Here's how the part is built. I have some questions about the finished solid (model axes, mm). Face numbers are marked on the shaded views. A direction names the side the tool comes from. Give positions to 0.01 mm unless a question says otherwise; leave off trailing zeros. Order: outer loops, then holes, each group sorted by start corner. A loop starts at its lowest first (then second) coordinate and runs counter-clockwise, first axis right, second up.
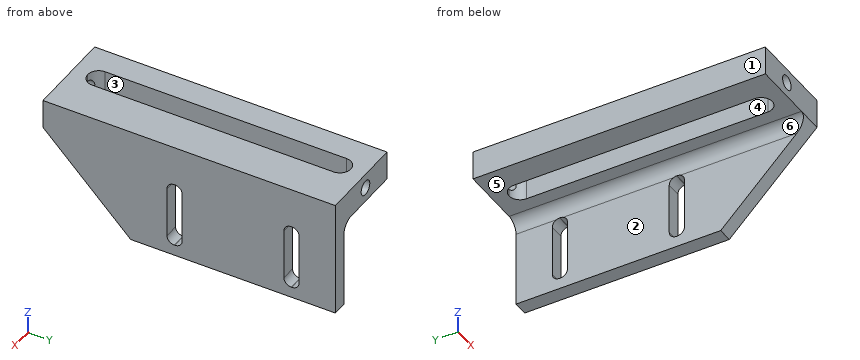
from build123d import *

# Parameters (mm, degrees)
F1_DEPTH  = 127
F2_R      = 5.08
F4_DEPTH  = 50.801
F5_R      = 3.175
F6_DEPTH  = 127.001
F8_DEPTH  = 38.101
F10_DEPTH = 38.101


with BuildPart() as f1:
    # F0 (on Front) → F1 (new body)
    with BuildSketch(Plane.XZ):
        Polygon((19.05, -25.4), (19.05, 25.4), (-19.05, 25.4), (-19.05, 12.7), (12.7, 12.7), (12.7, -25.4), align=None)
    extrude(amount=F1_DEPTH)

    # F2
    f2_edges = [f1.edges().sort_by_distance(p)[0] for p in [
        (12.7, -63.5, 12.7),
    ]]
    fillet(f2_edges, radius=F2_R)

    # F3 (on face) → F4 (cut, through all)
    with BuildSketch(Plane.XY.offset(25.4)):
        with BuildLine():
            Line((-3.1623, -6.35), (-3.1877, -6.35))
            ThreePointArc((-3.1877, -6.35), (-6.546316, -7.741184), (-7.9375, -11.0998))
            Line((-7.9375, -11.0998), (-7.9375, -115.9002))
            ThreePointArc((-7.9375, -115.9002), (-6.546316, -119.258816), (-3.1877, -120.65))
            Line((-3.1877, -120.65), (-3.1623, -120.65))
            ThreePointArc((-3.1623, -120.65), (0.196316, -119.258816), (1.5875, -115.9002))
            Line((1.5875, -115.9002), (1.5875, -11.0998))
            ThreePointArc((1.5875, -11.0998), (0.196316, -7.741184), (-3.1623, -6.35))
        make_face()
    extrude(amount=-F4_DEPTH, mode=Mode.SUBTRACT)

    # F5 (on face) → F6 (cut, through all)
    with BuildSketch(Plane.XZ.offset(127)):
        with Locations((-3.175, 19.05)):
            Circle(F5_R)
    extrude(amount=-F6_DEPTH, mode=Mode.SUBTRACT)

    # F7 (on face) → F8 (cut, through all)
    with BuildSketch(Plane.YZ.offset(19.05)):
        Polygon((-127, 12.7), (-127, -25.4), (-88.9, -25.4), align=None)
    extrude(amount=-F8_DEPTH, mode=Mode.SUBTRACT)

    # F9 (on face) → F10 (cut, through all)
    with BuildSketch(Plane.YZ.offset(19.05)):
        with BuildLine():
            ThreePointArc((-66.548, 4.7625), (-67.477936, 7.007564), (-69.723, 7.9375))
            Line((-69.723, 7.9375), (-69.977, 7.9375))
            ThreePointArc((-69.977, 7.9375), (-72.222064, 7.007564), (-73.152, 4.7625))
            Line((-73.152, 4.7625), (-73.152, -17.4625))
            ThreePointArc((-73.152, -17.4625), (-72.222064, -19.707564), (-69.977, -20.6375))
            Line((-69.977, -20.6375), (-69.723, -20.6375))
            ThreePointArc((-69.723, -20.6375), (-67.477936, -19.707564), (-66.548, -17.4625))
            Line((-66.548, -17.4625), (-66.548, 4.7625))
        make_face()
        with BuildLine():
            ThreePointArc((-15.748, 4.7625), (-16.677936, 7.007564), (-18.923, 7.9375))
            Line((-18.923, 7.9375), (-19.177, 7.9375))
            ThreePointArc((-19.177, 7.9375), (-21.422064, 7.007564), (-22.352, 4.7625))
            Line((-22.352, 4.7625), (-22.352, -17.4625))
            ThreePointArc((-22.352, -17.4625), (-21.422064, -19.707564), (-19.177, -20.6375))
            Line((-19.177, -20.6375), (-18.923, -20.6375))
            ThreePointArc((-18.923, -20.6375), (-16.677936, -19.707564), (-15.748, -17.4625))
            Line((-15.748, -17.4625), (-15.748, 4.7625))
        make_face()
    extrude(amount=-F10_DEPTH, mode=Mode.SUBTRACT)


solid = f1.part
Q1. If we section it at A-A on z = -8: List the corners of the cut face in (x, y) for me.
Filled sheet:
outline: (12.7, -106.3) - (19.05, -106.3) - (19.05, -73.15) - (12.7, -73.15) - close; (12.7, -66.55) - (19.05, -66.55) - (19.05, -22.35) - (12.7, -22.35) - close; (12.7, -15.75) - (19.05, -15.75) - (19.05, 0) - (12.7, 0) - close
Q2. If we section it at D-D on y = -56.5: List the corners of the cut face in (x, z) for me, plus the area to 3 significant figures.
Filled sheet:
outline: (-19.05, 12.7) - (-7.94, 12.7) - (-7.94, 25.4) - (-19.05, 25.4) - close; (1.59, 12.7) - (7.62, 12.7) arc R5.08 cw to (12.7, 7.62) - (12.7, -25.4) - (19.05, -25.4) - (19.05, 25.4) - (1.59, 25.4) - close
area: 610 mm2
Q3. If we section it at C-C on z = 19.05: List the corners of the cut face in (x, y) for me.
Filled sheet:
outline: (-19.05, -127) - (-6.35, -127) - (-6.35, -119.44) arc R4.75 cw to (-7.94, -115.9) - (-7.94, -11.1) arc R4.75 cw to (-6.35, -7.56) - (-6.35, 0) - (-19.05, 0) - close; (0, -127) - (19.05, -127) - (19.05, 0) - (0, 0) - (0, -7.56) arc R4.75 cw to (1.59, -11.1) - (1.59, -115.9) arc R4.75 cw to (0, -119.44) - close
Q4. I need wall thicknesses on L1, parallel to X at y = -51.5, z = 19.5; L2, parallel to Y at x = 15.5, z = -9; L3, parallel to X at y = -122, z = 19. Which ranges of each line are inside material? Lowest first, please.
Filled sheet:
L1: x = -19.05 to -7.94, 1.59 to 19.05
L2: y = -105.3 to -73.15, -66.55 to -22.35, -15.75 to 0
L3: x = -19.05 to -6.35, 0 to 19.05
Q5. Thinking about a two-plate mould opening in X: for the marked faces 4, 5 and 6, which applies, released by +X, released by -X, zero draft, split by the parting line, or undercut?
Filled sheet:
face 4: undercut
face 5: zero draft
face 6: released by -X
Q6. If we section it at B-B on y = -112.5: List the corners of the cut face in (x, z) for me.
Filled sheet:
outline: (-19.05, 12.7) - (-7.94, 12.7) - (-7.94, 25.4) - (-19.05, 25.4) - close; (1.59, 12.7) - (7.62, 12.7) arc R5.08 cw to (12.7, 7.62) - (12.7, -1.8) - (19.05, -1.8) - (19.05, 25.4) - (1.59, 25.4) - close
Q7. For the marked faces 1, 2 and 3, which set-ups out of +Z, -Z, +X, -X, +Y, -Y let a thin tool reach every point of the face, with its end or its side?
Filled sheet:
face 1: +Z, -Z, -X, +Y, -Y
face 2: -Z, -X, +Y, -Y
face 3: +Z, -Z
Q8. I'm going to push flat-ended pins straight in: P1, Ø4, axis at x = 7.5, y = -51, coming from the -Z side; P2, Ø5, axis at y = -34, z = -15, coming from the -X side; P3, Ø2, axis at x = -8, y = -74.5, coming from the -Z side. Where does each tip first touch, or does it pass through?
Filled sheet:
P1: stops at z = 12.34
P2: stops at x = 12.7
P3: stops at z = 12.7
